CAD build for the part. Positions are in the model's coordinates, mm. A direction names the side the tool comes from. Give positions to 0.01 mm unless a question says otherwise; leave off trailing zeros. Loops run counter-clockwise (first coordinate to the right, second up) from the corner with the lowest first, then second, coordinate; pieces in that order, holes last.
```python
from build123d import *

# Parameters (mm, degrees)
SKETCH_2_W          = 41
SKETCH_2_H          = 106
SKETCH_2_R          = 1.65
EXTRUDE_3_DEPTH     = 23
SKETCH_5_R          = 1.65
CUT_EXTRUDE_2_DEPTH = 113.169514575
SKETCH_6_W          = 41
SKETCH_6_H          = 106
EXTRUDE_4_DEPTH     = 3
CUT_EXTRUDE_START   = -2
SKETCH_7_W          = 10.5
SKETCH_7_H          = 10.5
SKETCH_7_W_2        = 10
SKETCH_7_H_2        = 10
CUT_EXTRUDE_3_DEPTH = 111.822870022
FILLET_1_R          = 8
FILLET_2_R          = 6
FILLET_3_R          = 3


with BuildPart() as part:
    # 草图2 → 凸台-拉伸3 (new body)
    with BuildSketch(Plane.XY):
        with Locations((17.5, 50)):
            Rectangle(SKETCH_2_W, SKETCH_2_H)
        Polygon((9, 0), (9, 9), (0, 9), (0, 91), (9, 91), (9, 100), (27, 100), (27, 92), (35, 92), (35, 9), (26, 9), (26, 0), align=None, mode=Mode.SUBTRACT)
        with Locations((4.5, 4.5)):
            Circle(SKETCH_2_R, mode=Mode.SUBTRACT)
        with Locations((4.5, 95.5)):
            Circle(SKETCH_2_R, mode=Mode.SUBTRACT)
        with Locations((30.5, 95.5)):
            Circle(SKETCH_2_R, mode=Mode.SUBTRACT)
    extrude(amount=EXTRUDE_3_DEPTH)

    # 草图5 → 切除-拉伸2 (cut, through all)
    with BuildSketch(Plane.XY.offset(23)):
        with Locations((30.5, 4.5)):
            Circle(SKETCH_5_R)
    extrude(amount=-CUT_EXTRUDE_2_DEPTH, mode=Mode.SUBTRACT)

    # 草图6 → 凸台-拉伸4 (add)
    with BuildSketch(Plane(origin=(0, 0, 0), x_dir=(-1, 0, 0), z_dir=(0, 0, -1))):
        with Locations((-17.5, 50)):
            Rectangle(SKETCH_6_W, SKETCH_6_H)
    extrude(amount=EXTRUDE_4_DEPTH)

    # 草图7 → 切除-拉伸3 (cut, through all)
    with BuildSketch(Plane.XY.offset(23).offset(CUT_EXTRUDE_START)):
        with Locations((2.25, 97.75)):
            Rectangle(SKETCH_7_W, SKETCH_7_H)
        with Locations((33, 98)):
            Rectangle(SKETCH_7_W_2, SKETCH_7_H_2)
        with Locations((2.25, 2.25)):
            Rectangle(SKETCH_7_W, SKETCH_7_H)
        with Locations((32.75, 2.25)):
            Rectangle(SKETCH_7_W, SKETCH_7_H)
    extrude(amount=-CUT_EXTRUDE_3_DEPTH, mode=Mode.SUBTRACT)

    # 圆角1
    fillet_1_edges = [part.edges().sort_by_distance(p)[0] for p in [
        (-3, -3, 22),
        (-3, 103, 22),
        (38, 103, 22),
        (38, -3, 22),
    ]]
    fillet(fillet_1_edges, radius=FILLET_1_R)

    # 圆角2
    fillet_2_edges = [part.edges().sort_by_distance(p)[0] for p in [
        (38, 50.25, -3),
        (-3, 50, -3),
    ]]
    fillet(fillet_2_edges, radius=FILLET_2_R)

    # 圆角3
    fillet_3_edges = [part.edges().sort_by_distance(p)[0] for p in [
        (17.5, -3, -3),
        (17.75, 103, -3),
        (27.5, -3, 9),
        (27.5, 2.25, -3),
        (7.5, 103, 9),
        (7.5, 97.75, -3),
        (28, 98, -3),
        (28, 103, 9),
        (7.5, 2.25, -3),
        (7.5, -3, 9),
        (29.75, 7.5, -3),
        (5.25, 7.5, -3),
        (5.25, 92.5, -3),
        (30, 93, -3),
        (-3, 92.5, 12),
        (-1.242640687, 92.5, -1.242640687),
        (-3, 7.5, 12),
        (-1.242640687, 7.5, -1.242640687),
        (38, 7.5, 12),
        (36.242640687, 7.5, -1.242640687),
        (38, 93, 12),
        (36.242640687, 93, -1.242640687),
    ]]
    fillet(fillet_3_edges, radius=FILLET_3_R)


solid = part.part
```
1. Drop flat-ended pins along their axis: pin 1 (2 mm diameter, centred on x = 4, z = 7, fed in from -Y); pin 2 (10 mm diameter, centred on x = 4, z = 9.5, fed in from -Y); pin 3 (4 mm diameter, centred on y = 69.5, z = 0.5, fed in from +X). Give the stop position or say it passes through.
Responses:
pin 1: stops at y = 7.5
pin 2: stops at y = -2.6
pin 3: stops at x = 37.98
2. Saw through at C-C, the plane x = 22. List the corners of the cut face in (y, z).
Responses:
outline: (-3, 0) arc R3 ccw to (0, -3) - (100, -3) arc R3 ccw to (103, 0) - (103, 23) - (100, 23) - (100, 0) - (0, 0) - (0, 23) - (-3, 23) - close
3. Saw through at B-B, the plane y = 42.5. List the corners of the cut face in (x, z).
Responses:
outline: (-3, 3) arc R6 ccw to (3, -3) - (32, -3) arc R6 ccw to (38, 3) - (38, 23) - (35, 23) - (35, 0) - (0, 0) - (0, 23) - (-3, 23) - close
4. Tool access for faces 5 (the face through (27.1, 96.04, -2.14)), 6 (the face through (29.03, 8.36, -2.1)), 7 (the face through (8.4, -2.14, 10.35)): list every direction of +Z, -Z, +X, -X, +Y, -Y with a clear straight run to the whole face (end or side of a thin tool).
Responses:
face 5: -Z, +X, +Y
face 6: -Z, +X, -Y
face 7: -Z, -X, -Y
5. Probe line 1 along Y through (x, z) = (4.5, 21.85); line 2 along X through (y, z) = (50.5, 10); line 3 along X through (y, z) = (3, 1). List the from-to ranges inside material, lowest first.
Responses:
line 1: y = -2.98 to 2.85, 6.15 to 9, 91 to 93.85, 97.15 to 102.98
line 2: x = -3 to 0, 35 to 38
line 3: x = 7.5 to 9, 26 to 27.5
6. Pull direction X, two halves, no side cores. Call faces 1 (the face through (0, 49, 11)), 2 (the face through (30.1, 93.9, 22)), 3 (the face through (-3, 49, 13)), 4 (the face through (5.86, 8.4, -2.14)): released by +X, released by -X, zero draft, split by the parting line, or undercut.
Responses:
face 1: undercut
face 2: undercut
face 3: released by -X
face 4: zero draft
